Autodesk Inventor part; units mm, degrees
ref_plane "YZ Plane" through (0, 0, 0) normal (1, 0, 0) x (0, 1, 0)
ref_plane "XZ Plane" through (0, 0, 0) normal (0, 1, 0) x (-1, 0, 0)
ref_plane "XY Plane" through (0, 0, 0) normal (0, 0, 1) x (1, 0, 0)
sketch "スケッチ1" plane through (0, 0, 0) normal (0, 1, 0) x (-1, 0, 0)
  line L0 (-15, -5) -> (15, -5)
  line L1 (15, -5) -> (15, 5)
  line L2 (15, 5) -> (-15, 5)
  line L3 (-15, 5) -> (-15, -5)
  line L4 (-15, -5) -> (15, 5) construction
  line L5 (15, -5) -> (-15, 5) construction
  point P0 (0, 0)
  dimension "d0" = 30
  dimension "d1" = 10
extrude "押し出し1" add sketch "スケッチ1" along normal blind 2
sketch "スケッチ2" plane through (15, 0, 5) normal (1, 0, 0) x (0, 0, -1)
  circle A0 centre (5, 7) radius 2.5
  circle A1 centre (5, 7) radius 5
  line L0 (0, 2) -> (10, 2)
  line L1 (10, 0) -> (10, 2)
  line L2 (0, 0) -> (0, 2)
  line L3 (0, 2) -> (0, 7)
  line L4 (10, 2) -> (10, 7)
  line L5 (0, 0) -> (10, 0)
  point P0 (5, 0)
  dimension "d4" = 5
extrude "押し出し2" add sketch "スケッチ2" along normal blind 5
mirror "ミラー1" about plane through (0, 0, 0) normal (1, 0, 0) of "押し出し2"
sketch "スケッチ3" plane through (20, 0, 5) normal (1, 0, 0) x (0, 0, -1)
  circle A0 centre (5, 7) radius 2.5
  point P0 (5, 0)
extrude "押し出し3" add sketch "スケッチ3" against normal up to surface (40 mm away)
properties part number "arm_base"
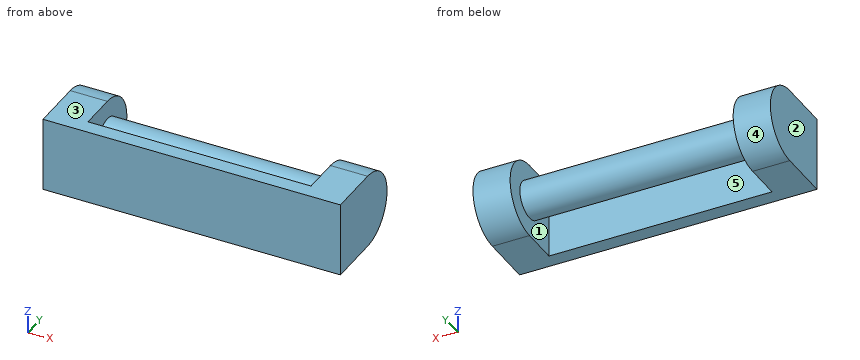
Part model, mm, in its own coordinate system. Face numbers are marked on the shaded views. A direction names the side the tool comes from. Give positions to 0.01 mm unless a question says otherwise; leave off trailing zeros. Write each loop counter-clockwise with the first axis right and the second up, starting at its lowest first coordinate (ties: lowest second). Pieces come first, ordered by that corner, then holes. Notation, with made-up numbers: M -5,70.25 L 20,70.25 A34 cw 20,102.25 Z; hole C 47,40.5 d1. An arc over 180 degrees is marked long. Use CSV: the item, a comma, the result in double quotes.
Item 1: Pull direction Y, two halves, no side cores. Call the marked faces 3, 4 and 5: +Y half, -Y half, draft (parallel to the pull), parting line (faces both ways), or undercut.
Taken from the geometry:
face 3,"draft"
face 4,"+Y half"
face 5,"undercut"
Item 2: Slice it at A-A on z = 0. Write the cut outline in (x, y).
Taken from the geometry:
outline,"M -20,0 L 20,0 L 20,12 L 15,12 L 15,9.5 L -15,9.5 L -15,12 L -20,12 Z; hole M -15,2 L 15,2 L 15,4.5 L -15,4.5 Z"
Item 3: Slice it at D-D on z = 3.25. Write the cut outline in (x, y).
Taken from the geometry:
outline,"M -20,0 L 20,0 L 20,10.8 L 15,10.8 L 15,2 L -15,2 L -15,10.8 L -20,10.8 Z"
Item 4: Pin check, flat tip, straight feed: P1, Ø1.5, axis at x = 11, y = 9, coming from the -Z side. Stop position of the tip, or through.
Taken from the geometry:
P1,"stops at z = -2.17"
Item 5: Drill centre lines: probe 1 along X at (y, z) = (9.25, 4); probe 2 along Y at (x, z) = (-7, 0); probe 3 along Y at (x, z) = (5, 1.5). Where is each one in solid material? Low to high.
Taken from the geometry:
probe 1,"x = -20 to -15, 15 to 20"
probe 2,"y = 0 to 2, 4.5 to 9.5"
probe 3,"y = 0 to 2, 5 to 9"
Item 6: Which spindle directions (+Z, -Z, +X, -X, +Y, -Y) get a long thin tool onto all of the face, cutting with end or side? Do the marked faces 1 and 2. Say none if no direction does.
Taken from the geometry:
face 1,"none"
face 2,"+Z, -Z, -X, +Y, -Y"
Item 7: Slice it at C-C on y = 11. Write the cut outline in (x, z).
Taken from the geometry:
outline,"M -20,-3 L -15,-3 L -15,3 L -20,3 Z; M 15,-3 L 20,-3 L 20,3 L 15,3 Z"
Item 8: Slice it at B-B on x = 12. Write the cut outline in (y, z), plus the area to 3 significant figures.
Taken from the geometry:
outline,"M 0,-5 L 2,-5 L 2,5 L 0,5 Z; C 7,0 d5"
area,"39.6 mm²"
